```python
from build123d import *

# Parameters (mm, degrees)
F0_W          = 6
F0_H          = 8
F1_DEPTH      = 4
F1_DEPTH_BACK = 4
F2_R          = 1
F3_DEPTH      = 8.001
F4_R          = 1
F5_DEPTH      = 6.001
F6_R          = 1.2
F7_DEPTH      = 4
F8_R          = 1.2
F9_DEPTH      = 3


with BuildPart() as f1:
    # F0 (on Front) → F1 (new body, two sides)
    with BuildSketch(Plane.XZ) as f1_sk:
        Rectangle(F0_W, F0_H)
    extrude(amount=F1_DEPTH)
    extrude(f1_sk.sketch, amount=-F1_DEPTH_BACK)

    # F2 (on face) → F3 (cut, through all)
    with BuildSketch(Plane.XZ.offset(4)):
        with Locations((0, 1.5)):
            Circle(F2_R)
    extrude(amount=-F3_DEPTH, mode=Mode.SUBTRACT)

    # F4 (on face) → F5 (cut, through all)
    with BuildSketch(Plane.YZ.offset(3)):
        with Locations((0, -1.5)):
            Circle(F4_R)
    extrude(amount=-F5_DEPTH, mode=Mode.SUBTRACT)

    # F6 (on face) → F7 (cut)
    with BuildSketch(Plane.XZ.offset(4)):
        with Locations((0, -1.5)):
            Circle(F6_R)
    extrude(amount=-F7_DEPTH, mode=Mode.SUBTRACT)

    # F8 (on face) → F9 (cut)
    with BuildSketch(Plane.YZ.offset(3)):
        with Locations((0, 1.5)):
            Circle(F8_R)
    extrude(amount=-F9_DEPTH, mode=Mode.SUBTRACT)


solid = f1.part
```
For this review, take the finished solid that the model builds, in its own axes (mm). A direction names the side the tool comes from. Round coordinates to 2 decimals unless told otherwise and drop trailing zeros. Write each loop counter-clockwise with the first axis right and the second up, starting at its lowest first coordinate (ties: lowest second). Pieces come first, ordered by that corner, then holes. Notation, with made-up numbers: (-37.5, 11) -> (-13.5, 11) arc R22 cw to (-13.5, 18) -> close; hole circle Ø7 at (0.5, -4). An arc over 180 degrees is marked (long way). One line per question, with ' | ' between items. Start each with the question number.
1) Machinability: for faces 5 (the cylindrical face through (1.854, 1.145, 1.86)), 6 (the flat face through (0, 0, 4)), 7 (the cylindrical face through (-1.2, -2.03, -1.45)), which of the approach directions +Z, -Z, +X, -X, +Y, -Y give a long, thin tool a straight path to every point of the face, cutting with its end or side? Answer none if there is none.
2) Add section A-A (y = 2). Write out the cut boundary in (x, z), and give its area (3 significant figures).
3) Add section C-C (x = -1.5). Write out the cut boundary in (y, z).
4) Add section B-B (z = 0.75). Write out the cut boundary in (x, y).
5) Add section D-D (y = -2). Write out the cut boundary in (x, z).
6) For pin 1 Ø1.8 at (y, z) = (0, -1.5) entering from +X, flat-tipped, find the tip position at first contact; note if it passes through.
7) Wall thickness on line 1 along Z through (x, y) = (0, -1); line 2 along Y through (x, z) = (-1.75, -2.25); line 3 along Z through (x, y) = (0.75, -2.5): over which ranges is each line inside the solid? List them lowest first.
8) Mouldability with a two-part tool opening along X and no side actions: class faces 1 (the flat face through (-3, 0, 0)), 2 (the flat face through (3, 0, 0)), 3 (the flat face through (0, -4, 0)), 4 (the cylindrical face through (-1, -0.1, 1.5)) as +X half, -X half, draft (parallel to the pull), parting line (faces both ways), or undercut.
Reported:
1) face 5: +X | face 6: +Z, +X, -X, +Y, -Y | face 7: -Y
2) outline: (-3, -4) -> (3, -4) -> (3, 4) -> (-3, 4) -> close; hole circle Ø2 at (0, 1.5) | area: 44.9 mm²
3) outline: (-4, -4) -> (4, -4) -> (4, 4) -> (-4, 4) -> close; hole circle Ø2 at (0, -1.5)
4) outline: (-3, -4) -> (-0.66, -4) -> (-0.66, 4) -> (-3, 4) -> close; (0.66, -4) -> (3, -4) -> (3, -0.94) -> (0.66, -0.94) -> close; (0.66, 0.94) -> (3, 0.94) -> (3, 4) -> (0.66, 4) -> close
5) outline: (-3, -4) -> (3, -4) -> (3, 4) -> (-3, 4) -> close; hole circle Ø2.4 at (0, -1.5); hole circle Ø2 at (0, 1.5)
6) pin 1: passes through
7) line 1: z = -4 to -2.7, -0.3 to 0.5, 2.5 to 4 | line 2: y = -4 to -0.66, 0.66 to 4 | line 3: z = -4 to -2.44, -0.56 to 0.84, 2.16 to 4
8) face 1: -X half | face 2: +X half | face 3: draft | face 4: undercut
